Could you check a few things on this drawing? It's one solid part, dimensions in mm from its lowest x, y, z. A direction names the side the tool comes from. Round coordinates to 2 decimals unless told otherwise and drop trailing zeros. Loops run counter-clockwise (first coordinate to the right, second up) from the corner with the lowest first, then second, coordinate; pieces in that order, holes last. Notation, with made-up numbers: M -34,-4 L -8,-4 A35 cw -8,33 Z; hole C 44.25,-30 d1. An arc over 180 degrees is marked long. Return JSON: item names as keys, results as strings.
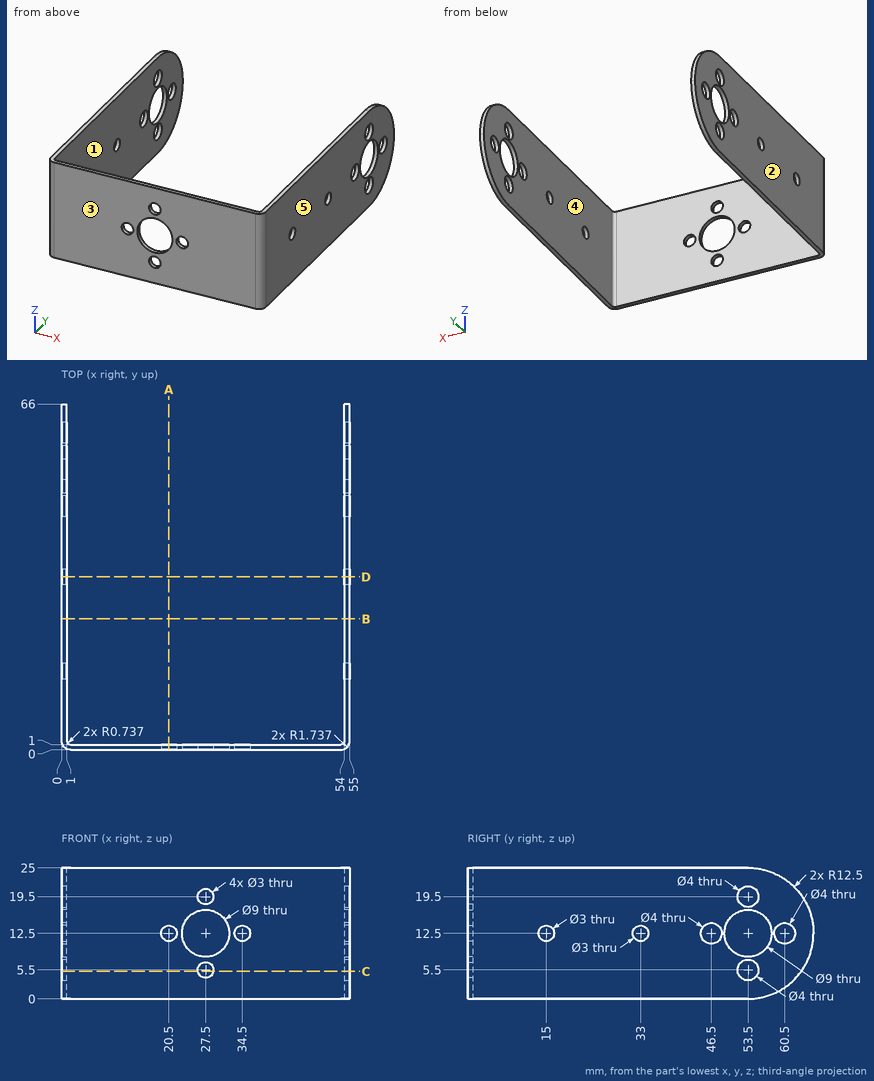
Q1. Suppose I cut it at A-A, the plane x = 20.5. Please give me the cut outline in (y, z), plus the area to 3 significant figures.
Results:
{"outline": "M 0,0 L 1,0 L 1,11 L 0,11 Z; M 0,14 L 1,14 L 1,25 L 0,25 Z", "area": "22.0 mm2"}
Q2. On a 3-axis mill with a long thin cutter (end or side, diameter ignored), from which of +Z, -Z, +X, -X, +Y, -Y can I reach the whole of each face in a straight line? I mean the marked faces 4 and 5. Say none if no direction works.
Results:
{"face 4": "+Z, -Z, +Y", "face 5": "+Z, -Z, +X, +Y, -Y"}
Q3. Suppose I cut it at C-C, the plane z = 5.25. Please give me the cut outline in (x, y) (1 decimal).
Results:
{"outline": "M 0,1.7 A1.7 ccw 1.7,0 L 26,0 L 26,1 L 1.7,1 A0.7 cw 1,1.7 L 1,51.5 L 0,51.5 Z; M 0,55.5 L 1,55.5 L 1,63.7 L 0,63.7 Z; M 29,0 L 53.3,0 A1.7 ccw 55,1.7 L 55,51.5 L 54,51.5 L 54,1.7 A0.7 cw 53.3,1 L 29,1 Z; M 54,55.5 L 55,55.5 L 55,63.7 L 54,63.7 Z"}
Q4. I'm going to push flat-ended pins straight in: pin 1 Ø3.5 at (y, z) = (53.5, 19.5) entering from -X; pin 2 Ø1 at (x, z) = (44.5, 16.5) entering from +Y. Where does each tip first touch, or does it pass through?
Results:
{"pin 1": "passes through", "pin 2": "stops at y = 1"}
Q5. Thinking about a two-plate mould opening in X: for the marked faces 1, 2 and 3, which applies, pulls with the +X half, pulls with the -X half, needs draft (parallel to the pull), parting line crosses it, or undercut?
Results:
{"face 1": "undercut", "face 2": "pulls with the -X half", "face 3": "needs draft"}
Q6. Suppose I cut it at B-B, the plane y = 25. Please give me the cut outline in (x, z).
Results:
{"outline": "M 0,0 L 1,0 L 1,25 L 0,25 Z; M 54,0 L 55,0 L 55,25 L 54,25 Z"}
Q7. Suppose I cut it at D-D, the plane y = 33. Please give me the cut outline in (x, z).
Results:
{"outline": "M 0,0 L 1,0 L 1,11 L 0,11 Z; M 0,14 L 1,14 L 1,25 L 0,25 Z; M 54,0 L 55,0 L 55,11 L 54,11 Z; M 54,14 L 55,14 L 55,25 L 54,25 Z"}
Q8. If I drill on line 1 along Z through (x, y) = (54.85, 53.5); line 2 along X through (y, z) = (10, 23); line 3 along Z through (x, y) = (54.4, 46.5), over which ranges is the centre line in solid material (lowest first)?
Results:
{"line 1": "z = 0 to 3.5, 7.5 to 8, 17 to 17.5, 21.5 to 25", "line 2": "x = 0 to 1, 54 to 55", "line 3": "z = 0 to 10.5, 14.5 to 25"}
